from build123d import *

# Parameters (mm, degrees)
F0_W     = 35
F0_H     = 350
F0_R     = 5
F1_DEPTH = 15
F2_W     = 15
F2_H     = 350
F3_DEPTH = 109
F5_DEPTH = 15
F7_DEPTH = 5


with BuildPart() as f1:
    # F0 (on Top) → F1 (new body)
    with BuildSketch(Plane.XY):
        with Locations((-57.72887, 129.090141)):
            Rectangle(F0_W, F0_H)
        with Locations((-50.22887, -15.909859)):
            Circle(F0_R, mode=Mode.SUBTRACT)
        with Locations((-50.22887, 129.090141)):
            Circle(F0_R, mode=Mode.SUBTRACT)
        with Locations((-50.22887, 274.090141)):
            Circle(F0_R, mode=Mode.SUBTRACT)
    extrude(amount=F1_DEPTH)

    # F2 (on face) → F3 (join)
    with BuildSketch(Plane.XY.offset(15)):
        with Locations((-67.72887, 129.090141)):
            Rectangle(F2_W, F2_H)
    extrude(amount=F3_DEPTH)

    # F4 (on face) → F5 (join)
    with BuildSketch(Plane.YZ.offset(-60.22887)):
        Polygon((-45.909859, 332.642), (-45.909859, 124), (304.090141, 124), align=None)
    extrude(amount=-F5_DEPTH)

    # F6 (on face) → F7 (cut)
    with BuildSketch(Plane(origin=(-75.22887, 0, 0), x_dir=(0, -1, 0), z_dir=(-1, 0, 0))):
        Polygon((45.909859, 320.417912), (45.909859, 326.821006), (-297.235123, 122.265419), (-294.418886, 117.54114), align=None)
    extrude(amount=-F7_DEPTH, mode=Mode.SUBTRACT)


solid = f1.part
For this review, take the finished solid that the model builds, in its own axes (mm). A direction names the side the tool comes from. Give positions to 0.01 mm unless a question says otherwise; leave off trailing zeros. Loops run counter-clockwise (first coordinate to the right, second up) from the corner with the lowest first, then second, coordinate; pieces in that order, holes last.
Item 1: Take a section at B-B, the plane z = 292.5. State the section outline as (x, y) points, and give its area (3 significant figures).
Item 2: Tool access review of faces 5 (the flat face through (-55, 132, 15)), 6 (the cylindrical face through (-47.922, 269.654, 7.395)), 7 (the flat face through (-72.764, 123.261, 225.975)): name each direction out of +Z, -Z, +X, -X, +Y, -Y from which nothing blocks a thin tool from reaching the whole face with its end or side.
Item 3: Draft analysis for pull direction X (two halves, no side actions). For faces 1 (the cylindrical face through (-50.88, 134.048, 7.395)), 2 (the cylindrical face through (-45.46, -14.41, 7.4)), 3 (the flat face through (-60.229, 88, 141)), 4 (the flat face through (-58, 132, 0)), state which applies: +X half, -X half, draft (parallel to the pull), parting line (faces both ways), or undercut.
Item 4: Take a section at D-D, the plane z = 223. State the section outline as (x, y) points.
Item 5: Take a section at C-C, the plane y = 53.5. State the section outline as (x, z) points, and give its area (3 significant figures).
Item 6: Take a section at A-A, the plane x = -49.5. State the section outline as (y, z) points, and give its area (3 significant figures).
Item 7: For line 1 along X through (y, z) = (120, 109.5); line 2 along Z through (x, y) = (-56.5, 134.5); line 3 along Z through (x, y) = (-72, 244), list the stretches that pass through material, from the lowest coordinate up.
Item 8: Insertion check: pin 1 (10 mm diameter, centred on x = -47.5, y = 52.5, fed in from +Z); pin 2 (8 mm diameter, centred on x = -64, z = 187, fed in from +Y); pin 3 (9 mm diameter, centred on x = -50.23, y = -15.91, fed in from +Z). Each pin has a flat end and moves straight along its axis. Give the tip position at first contact, or say it passes through.
Calculated:
1. outline: (-75.23, -45.91) - (-60.23, -45.91) - (-60.23, 21.43) - (-75.23, 21.43) - (-75.23, 11.66) - (-70.23, 11.66) - (-70.23, 0.92) - (-75.23, 0.92) - close
1. area: 956 mm2
2. face 5: +Z, +X, +Y, -Y
2. face 6: +Z, -Z
2. face 7: -X
3. face 1: undercut
3. face 2: undercut
3. face 3: +X half
3. face 4: draft
4. outline: (-75.23, -45.91) - (-60.23, -45.91) - (-60.23, 138.02) - (-75.23, 138.02) - (-75.23, 128.25) - (-70.23, 128.25) - (-70.23, 117.51) - (-75.23, 117.51) - close
5. outline: (-75.23, 0) - (-40.23, 0) - (-40.23, 15) - (-60.23, 15) - (-60.23, 273.38) - (-75.23, 273.38) - (-75.23, 267.56) - (-70.23, 267.56) - (-70.23, 261.16) - (-75.23, 261.16) - close
5. area: 4,370 mm2
6. outline: (-45.91, 0) - (-20.86, 0) - (-20.86, 15) - (-45.91, 15) - close; (-10.96, 0) - (124.14, 0) - (124.14, 15) - (-10.96, 15) - close; (134.04, 0) - (269.14, 0) - (269.14, 15) - (134.04, 15) - close; (279.04, 0) - (304.09, 0) - (304.09, 15) - (279.04, 15) - close
6. area: 4,800 mm2
7. line 1: x = -75.23 to -60.23
7. line 2: z = 0 to 15
7. line 3: z = 0 to 147.6, 154 to 159.82
8. pin 1: stops at z = 15
8. pin 2: stops at y = 205.12
8. pin 3: passes through
